CAD build for the part. Positions are in the model's coordinates, mm. A direction names the side the tool comes from. Coordinates: 2 decimals unless noted, no trailing zeros. Loops run counter-clockwise (first coordinate to the right, second up) from the corner with the lowest first, then second, coordinate; pieces in that order, holes last. Notation, with made-up numbers: (27, 31) -> (35, 31) arc R11 ccw to (35, 46) -> close; hole circle Ø8 at (23.5, 41.5). An arc over 180 degrees is marked (long way). Write each question's results on one line, items separated by ' | '.
from build123d import *

# Parameters (mm, degrees)
SKETCH1_R           = 4
BOSS_EXTRUDE1_DEPTH = 5
FILLET1_R           = 10
SCALE1_SCALE        = 0.5


with BuildPart() as part:
    # Sketch1 → Boss-Extrude1 (new body)
    with BuildSketch(Plane(origin=(0, 0, 0), x_dir=(1, 0, 0), z_dir=(0, 1, 0))):
        with BuildLine():
            Line((39.07179677, -4), (-39.07179677, -4))
            ThreePointArc((-39.07179677, -4), (-54, 0), (-39.07179677, 4))
            Line((-39.07179677, 4), (39.07179677, 4))
            ThreePointArc((39.07179677, 4), (54, 0), (39.07179677, -4))
        make_face()
        with Locations((-46, 0)):
            Circle(SKETCH1_R, mode=Mode.SUBTRACT)
        with Locations((46, 0)):
            Circle(SKETCH1_R, mode=Mode.SUBTRACT)
    extrude(amount=BOSS_EXTRUDE1_DEPTH)

    # Fillet1
    fillet1_edges = [part.edges().sort_by_distance(p)[0] for p in [
        (-39.07179677, 2.5, -4),
        (39.07179677, 2.5, -4),
        (39.07179677, 2.5, 4),
        (-39.07179677, 2.5, 4),
    ]]
    fillet(fillet1_edges, radius=FILLET1_R)


with BuildPart() as part_1:
    # Scale1: scaled about (0, 2.5, 0)
    add(part.part.scale(SCALE1_SCALE).moved(Location((0, 1.25, 0))))


solid = part_1.part
1) Slice it at A-A (z = 0). Write the cut outline in (x, y).
Outcome:
outline: (-27, 1.25) -> (-25, 1.25) -> (-25, 3.75) -> (-27, 3.75) -> close; (-21, 1.25) -> (21, 1.25) -> (21, 3.75) -> (-21, 3.75) -> close; (25, 1.25) -> (27, 1.25) -> (27, 3.75) -> (25, 3.75) -> close
2) Which spindle directions (+Z, -Z, +X, -X, +Y, -Y) get a long thin tool onto all of the face, cutting with end or side? Do faces 3 (the cylindrical face through (21, 2, 0)), 4 (the flat face through (0, 2, 2)), 5 (the cylindrical face through (19.032, 2.518, -2.294)). Say none if no direction does.
Outcome:
face 3: +Y, -Y | face 4: +Z, +Y, -Y | face 5: -Z, +Y, -Y
3) Slice it at C-C (y = 2.4). Write the cut outline in (x, z), then the cut area to 3 significant figures.
Outcome:
outline: (-20.49, -3.11) arc R5 cw to (-17.34, -2) -> (17.34, -2) arc R5 cw to (20.49, -3.11) arc R4 ccw (long way) to (20.49, 3.11) arc R5 cw to (17.34, 2) -> (-17.34, 2) arc R5 cw to (-20.49, 3.11) arc R4 ccw (long way) to start; hole circle Ø4 at (-23, 0); hole circle Ø4 at (23, 0) | area: 231 mm^2
4) Pin check, flat tips, straight feed: pin 1 (1.5 mm diameter, centred on y = 2.5, z = 2, fed in from +X); pin 2 (1.5 mm diameter, centred on x = -8.5, y = 2, fed in from +Z); pin 3 (0.8 mm diameter, centred on x = -8, y = 3, fed in from -Z). Stop position of each tip, or through.
Outcome:
pin 1: stops at x = 26.8 | pin 2: stops at z = 2 | pin 3: stops at z = -2
5) Two-plate mould, pull along X, no slides. Class faces 1 (the cylindrical face through (-18.99, 2.52, 2.28)), 2 (the flat face through (0, 1.25, 0)): pulls with the +X half, pulls with the -X half, needs draft (parallel to the pull), parting line crosses it, or undercut.
Outcome:
face 1: undercut | face 2: needs draft
6) Slice it at B-B (x = 23). Write the cut outline in (y, z), then the cut area to 4 significant figures.
Outcome:
outline: (1.25, -4) -> (3.75, -4) -> (3.75, -2) -> (1.25, -2) -> close; (1.25, 2) -> (3.75, 2) -> (3.75, 4) -> (1.25, 4) -> close | area: 10.00 mm^2
7) Slice it at D-D (x = -2.5). Write the cut outline in (y, z), then the cut area to 3 significant figures.
Outcome:
outline: (1.25, -2) -> (3.75, -2) -> (3.75, 2) -> (1.25, 2) -> close | area: 10.0 mm^2
8) Drill centre lines: L1, parallel to X at y = 2.8, z = 0; L2, parallel to Z at x = -23, y = 2.6; L3, parallel to X at y = 3.2, z = 1. Where is each one in solid material? Low to high. Write a range as from..to.
Outcome:
L1: x = -27..-25, -21..21, 25..27 | L2: z = -4..-2, 2..4 | L3: x = -26.87..-24.73, -21.27..21.27, 24.73..26.87
